```python
from build123d import *

# Parameters (mm, degrees)
SKETCH1_W           = 60
SKETCH1_H           = 60.2
BOSS_EXTRUDE1_DEPTH = 30.7
BOSS_EXTRUDE2_START = -15
BOSS_EXTRUDE2_DEPTH = 2
SKETCH3_R           = 3
BOSS_EXTRUDE3_DEPTH = 7
CHAMFER1_SIZE       = 10
SKETCH5_R           = 7.5
SKETCH5_R_2         = 3
BOSS_EXTRUDE4_DEPTH = 2
FILLET1_R           = 1
FILLET2_R           = 1
SKETCH6_W           = 28.7
SKETCH6_H           = 12.142135624
BOSS_EXTRUDE5_DEPTH = 1
FILLET3_R           = 1


with BuildPart() as part:
    # Sketch1 → Boss-Extrude1 (new body)
    with BuildSketch(Plane.XY):
        Rectangle(SKETCH1_W, SKETCH1_H)
    extrude(amount=BOSS_EXTRUDE1_DEPTH)

    # Sketch2 → Boss-Extrude2 (add)
    with BuildSketch(Plane(origin=(0, 30.1, 0), x_dir=(1, 0, 0), z_dir=(0, 1, 0)).offset(BOSS_EXTRUDE2_START)):
        with BuildLine():
            Line((-35.224448097, 0), (35.224448097, 0))
            Line((35.224448097, 0), (35.224448097, -5.886945825))
            ThreePointArc((35.224448097, -5.886945825), (31.5, -6.9), (35.224448097, -7.913054175))
            Line((35.224448097, -7.913054175), (35.224448097, -22.786945825))
            ThreePointArc((35.224448097, -22.786945825), (31.5, -23.8), (35.224448097, -24.813054175))
            Line((35.224448097, -24.813054175), (35.224448097, -30.7))
            Line((35.224448097, -30.7), (-35.224448097, -30.7))
            Line((-35.224448097, -30.7), (-35.224448097, -24.813054175))
            ThreePointArc((-35.224448097, -24.813054175), (-31.5, -23.8), (-35.224448097, -22.786945825))
            Line((-35.224448097, -22.786945825), (-35.224448097, -7.913054175))
            ThreePointArc((-35.224448097, -7.913054175), (-31.5, -6.9), (-35.224448097, -5.886945825))
            Line((-35.224448097, -5.886945825), (-35.224448097, 0))
        make_face()
    extrude(amount=BOSS_EXTRUDE2_DEPTH)

    # Sketch3 → Boss-Extrude3 (add)
    with BuildSketch(Plane(origin=(0, 30.1, 0), x_dir=(1, 0, 0), z_dir=(0, 1, 0))):
        with Locations(Location((-18, -15.35, 0), (0, 0, 90))):
            Circle(SKETCH3_R)
    extrude(amount=BOSS_EXTRUDE3_DEPTH)

    # Chamfer1
    chamfer1_edges = [part.edges().sort_by_distance(p)[0] for p in [
        (30, 30.1, 15.35),
    ]]
    chamfer(chamfer1_edges, length=CHAMFER1_SIZE)

    # Sketch5 → Boss-Extrude4 (add)
    with BuildSketch(Plane(origin=(0, 30.1, 0), x_dir=(1, 0, 0), z_dir=(0, 1, 0))):
        with Locations(Location((-18, -15.35, 0), (0, 0, 90))):
            Circle(SKETCH5_R)
        with Locations(Location((-18, -15.35, 0), (0, 0, 270))):
            Circle(SKETCH5_R_2, mode=Mode.SUBTRACT)
    extrude(amount=BOSS_EXTRUDE4_DEPTH)

    # Fillet1
    fillet1_edges = [part.edges().sort_by_distance(p)[0] for p in [
        (-18, 32.1, 22.85),
    ]]
    fillet(fillet1_edges, radius=FILLET1_R)

    # Fillet2
    fillet2_edges = [part.edges().sort_by_distance(p)[0] for p in [
        (0, -30.1, 30.7),
        (0, -30.1, 0),
        (30, -30.1, 15.35),
        (-30, -30.1, 15.35),
    ]]
    fillet(fillet2_edges, radius=FILLET2_R)

    # Sketch6 → Boss-Extrude5 (add)
    with BuildSketch(Plane(origin=(25.05, 25.05, 0), x_dir=(0, 0, -1), z_dir=(0.707106781186549, 0.707106781186546, 0))):
        with Locations((-15.35, 0.070710678)):
            Rectangle(SKETCH6_W, SKETCH6_H)
    extrude(amount=BOSS_EXTRUDE5_DEPTH)

    # Fillet3
    fillet3_edges = [part.edges().sort_by_distance(p)[0] for p in [
        (25.707106781, 25.807106781, 1),
        (30, 21.514213562, 15.35),
        (25.707106781, 25.807106781, 29.7),
        (21.414213562, 30.1, 15.35),
    ]]
    fillet(fillet3_edges, radius=FILLET3_R - 0.0001)  # a hair under: the kernel refuses the full size


solid = part.part
```
Could you check a few things on this model? Use its own coordinates, in mm. A direction names the side the tool comes from. Coordinates: 2 decimals unless noted, no trailing zeros. Write each loop counter-clockwise with the first axis right and the second up, starting at its lowest first coordinate (ties: lowest second). Pieces come first, ordered by that corner, then holes. Notation, with made-up numbers: (21, 76.25) -> (41, 76.25) arc R10 ccw to (41, 84.25) -> close; hole circle Ø11 at (72.5, 42). An arc over 180 degrees is marked (long way). One line per question, with ' | ' between items. Start each with the question number.
1. Please list where these lines run through material, in increasing order: line 1 along Z through (x, y) = (-33.5, 16.3); line 2 along Y through (x, z) = (-10, 6); line 3 along X through (y, z) = (15.9, 6.9).
2. If we section it at A-A (x = 33.5): Please give me the cut outline in (y, z).
3. For faces 1 (the face through (25.434, 25.655, 29.415)), 2 (the face through (-16.175, 34.565, 17.731)), 3 (the face through (-30, 24, 15)), 4 (the face through (25.657, 25.857, 15.537)), 5 (the face through (-33, 15.1, 15)), which set-ups out of +Z, -Z, +X, -X, +Y, -Y let a thin tool reach every point of the face, with its end or its side?
4. If we section it at D-D (y = -23): Please give me the cut outline in (x, z), and give its area (3 significant figures).
5. Will these pins go through, and if not, where does the flat tip stop? P1, Ø3, axis at x = 33.5, z = 6.9, coming from the -Y side; P2, Ø2.5, axis at x = 33.5, z = 21.5, coming from the -Y side; P3, Ø1, axis at y = -5.5, z = 18, coming from the -X side; P4, Ø9, axis at x = -9, z = 13, coming from the +Y side.
6. Thinking about a two-plate mould opening in X: for faces 6 (the face through (-31.5, 16.09, 23.87)), 7 (the face through (0, -30.1, 15)), 8 (the face through (30, 19, 15)), which applies, pulls with the +X half, pulls with the -X half, needs draft (parallel to the pull), parting line crosses it, or undercut?
7. If we section it at B-B (x = -18): Please give me the cut outline in (y, z).
Return value:
1) line 1: z = 0 to 4.9, 8.9 to 21.8, 25.8 to 30.7 | line 2: y = -30.1 to 30.1 | line 3: x = -31.5 to 31.5
2) outline: (15.1, 0) -> (17.1, 0) -> (17.1, 4.9) -> (15.1, 4.9) -> close; (15.1, 8.9) -> (17.1, 8.9) -> (17.1, 21.8) -> (15.1, 21.8) -> close; (15.1, 25.8) -> (17.1, 25.8) -> (17.1, 30.7) -> (15.1, 30.7) -> close
3) face 1: +Z, +X, +Y | face 2: +Y | face 3: +Z, -Z, -X, +Y | face 4: +Z, -Z, +X, +Y | face 5: +Z, -Z, -X, -Y
4) outline: (-30, 0) -> (30, 0) -> (30, 30.7) -> (-30, 30.7) -> close | area: 1,840 mm²
5) P1: passes through | P2: stops at y = 15.1 | P3: stops at x = -30 | P4: stops at y = 32.1
6) face 6: undercut | face 7: needs draft | face 8: pulls with the +X half
7) outline: (-30.1, 1) arc R1 ccw to (-29.1, 0) -> (30.1, 0) -> (30.1, 7.85) -> (31.1, 7.85) arc R1 ccw to (32.1, 8.85) -> (32.1, 12.35) -> (37.1, 12.35) -> (37.1, 18.35) -> (32.1, 18.35) -> (32.1, 21.85) arc R1 ccw to (31.1, 22.85) -> (30.1, 22.85) -> (30.1, 30.7) -> (-29.1, 30.7) arc R1 ccw to (-30.1, 29.7) -> close
